Geometry: see drawing. Coordinates: mm, zero at the bounding-box minimum. A direction names the side the tool comes from. Coordinates: 2 decimals unless noted, no trailing zeros. Write each loop counter-clockwise with the first axis right and the second up, starting at its lowest first coordinate (ties: lowest second). Pieces come first, ordered by that corner, then holes.
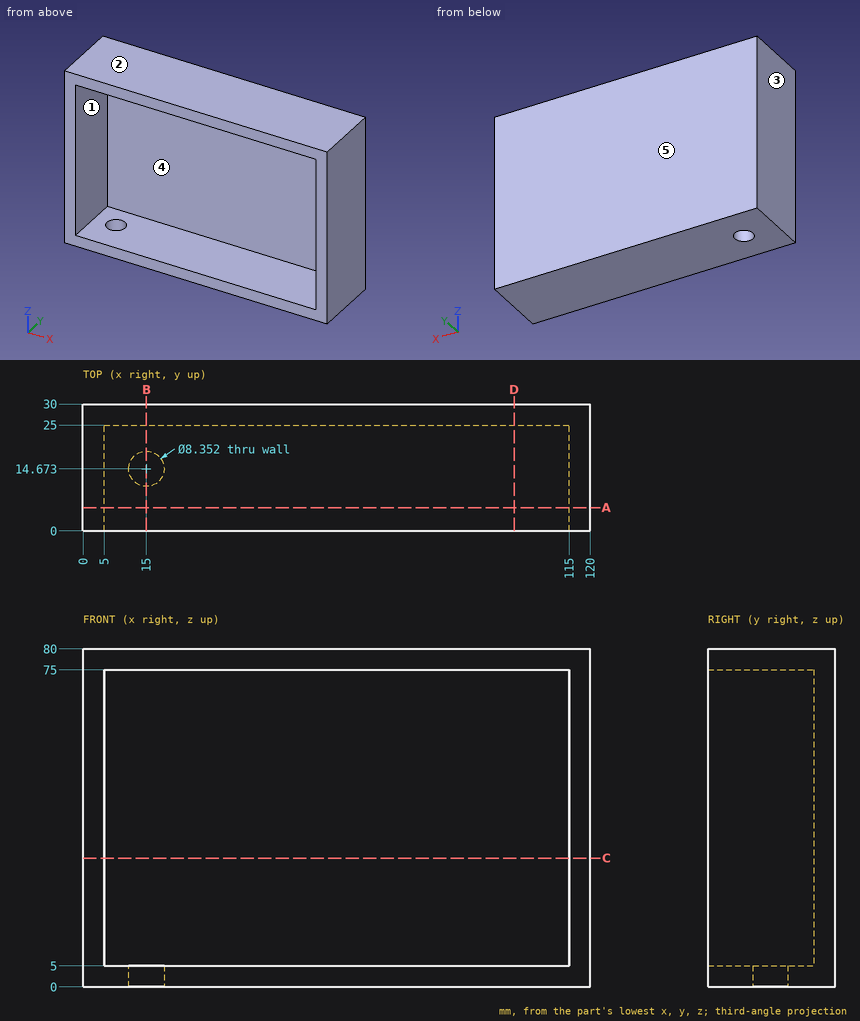
Item 1: Section A-A, the plane y = 5.5. Output: boundary loops of the cut face in (x, z).
Derived:
outline: (0, 0) - (120, 0) - (120, 80) - (0, 80) - close; hole (5, 5) - (115, 5) - (115, 75) - (5, 75) - close
Item 2: Set-up query: the marked faces 1 and 2. Return all of +Z, -Z, +X, -X, +Y, -Y with unobstructed straight access to the full face (end or side cutting, diameter ignored); none if empty.
Derived:
face 1: -Y
face 2: +Z, +X, -X, +Y, -Y
Item 3: Section C-C, the plane z = 30.5. Output: boundary loops of the cut face in (x, y).
Derived:
outline: (0, 0) - (5, 0) - (5, 25) - (115, 25) - (115, 0) - (120, 0) - (120, 30) - (0, 30) - close
Item 4: Section D-D, the plane x = 102. Output: boundary loops of the cut face in (y, z), plus the area to 3 significant figures.
Derived:
outline: (0, 0) - (30, 0) - (30, 80) - (0, 80) - (0, 75) - (25, 75) - (25, 5) - (0, 5) - close
area: 650 mm2
Item 5: Pull-direction query (X, two-part tool) for the marked faces 3, 4 and 5; classes: released by +X, released by -X, zero draft, split by the parting line, or undercut.
Derived:
face 3: released by -X
face 4: undercut
face 5: zero draft
Item 6: Section B-B, the plane x = 15. Output: boundary loops of the cut face in (y, z).
Derived:
outline: (0, 0) - (10.5, 0) - (10.5, 5) - (0, 5) - close; (0, 75) - (25, 75) - (25, 5) - (18.85, 5) - (18.85, 0) - (30, 0) - (30, 80) - (0, 80) - close
Item 7: Pin query (flat end, axial travel): pin 1 (2 mm diameter, centred on x = 39, z = 53, fed in from -Y). Return the tip coordinate at first contact, or that it passes through.
Derived:
pin 1: stops at y = 25
Item 8: Material intervals for probe 1 along Y at (x, z) = (15, 3.55); probe 2 along X at (y, z) = (24, 21.5); probe 3 along Z at (x, y) = (69.5, 19.75), sorted ascending.
Derived:
probe 1: y = 0 to 10.5, 18.85 to 30
probe 2: x = 0 to 5, 115 to 120
probe 3: z = 0 to 5, 75 to 80
